Part model, mm, in its own coordinate system. A direction names the side the tool comes from. Coordinates: 2 decimals unless noted, no trailing zeros. Write each loop counter-clockwise with the first axis right and the second up, starting at its lowest first coordinate (ties: lowest second). Pieces come first, ordered by that corner, then holes. Notation, with made-up numbers: (24.5, 6) - (58.5, 6) arc R23 cw to (58.5, 29) - close; hole circle Ø1 at (30, 70.5). An arc over 180 degrees is marked (long way). Use a Markdown table: item, result.
```python
from build123d import *

# Parameters (mm, degrees)
SKETCH_W               = 265
SKETCH_H               = 132.5
PAD_DEPTH              = 23
SKETCH001_W            = 249
SKETCH001_H            = 124.5
POCKET_DEPTH           = 2
SKETCH002_W            = 30
SKETCH002_H            = 30
PAD001_DEPTH           = 2
LINEARPATTERN_COUNT    = 8
LINEARPATTERN_PITCH    = 31
CHAMFER_SIZE           = 3
SKETCH003_W            = 31.42
SKETCH003_H            = 15.71
POCKET001_DEPTH        = 4.8
SKETCH004_W            = 255
SKETCH004_H            = 114.5
POCKET002_DEPTH        = 19
SKETCH005_R            = 7.6
POCKET003_DEPTH        = 2
LINEARPATTERN001_COUNT = 8
LINEARPATTERN001_PITCH = 32.142857
SKETCH006_R            = 7.6
POCKET004_DEPTH        = 2
LINEARPATTERN002_COUNT = 9
LINEARPATTERN002_PITCH = 28.125
SKETCH007_R            = 4.125
SKETCH007_R_2          = 4.025
POCKET005_DEPTH        = 1.8


with BuildPart() as part:
    # Sketch → Pad (new body)
    with BuildSketch(Plane.XY):
        with Locations((0, 66.25)):
            Rectangle(SKETCH_W, SKETCH_H)
    extrude(amount=PAD_DEPTH)

    # Sketch001 (on Face5 of Pad) → Pocket (cut)
    with BuildSketch(Plane(origin=(0, 0, 0), x_dir=(1, 0, 0), z_dir=(0, 0, -1))):
        with Locations((0, -62.25)):
            Rectangle(SKETCH001_W, SKETCH001_H)
    extrude(amount=-POCKET_DEPTH, mode=Mode.SUBTRACT)

    # Sketch002 (on Face10 of Pocket) → Pad001 (join)
    with BuildSketch(Plane(origin=(0, 0, 2), x_dir=(1, 0, 0), z_dir=(0, 0, -1))):
        with Locations((-108.5, -15.5)):
            Rectangle(SKETCH002_W, SKETCH002_H)
        with Locations((-108.5, -46.5)):
            Rectangle(SKETCH002_W, SKETCH002_H)
        with Locations((-108.5, -77.5)):
            Rectangle(SKETCH002_W, SKETCH002_H)
        with Locations((-108.5, -108.5)):
            Rectangle(SKETCH002_W, SKETCH002_H)
    pad001 = extrude(amount=PAD001_DEPTH)

    # LinearPattern: Pad001 ×8
    with Locations(*[(i * LINEARPATTERN_PITCH, 0, 0) for i in range(1, LINEARPATTERN_COUNT)]):
        add(pad001)

    # Chamfer
    chamfer_edges = [part.edges().sort_by_distance(p)[0] for p in [
        (-132.5, 66.25, 0),
        (0, 132.5, 0),
        (132.5, 66.25, 0),
    ]]
    chamfer(chamfer_edges, length=CHAMFER_SIZE)

    # Sketch003 (on Face6 of Chamfer) → Pocket001 (cut)
    with BuildSketch(Plane.XZ):
        with Locations((-86.79, 15.145)):
            Rectangle(SKETCH003_W, SKETCH003_H)
        with Locations((86.79, 15.145)):
            Rectangle(SKETCH003_W, SKETCH003_H)
    extrude(amount=-POCKET001_DEPTH, mode=Mode.SUBTRACT)

    # Sketch004 (on Face4 of Pocket001) → Pocket002 (cut)
    with BuildSketch(Plane.XY.offset(23)):
        with Locations((0, 65.25)):
            Rectangle(SKETCH004_W, SKETCH004_H)
    extrude(amount=-POCKET002_DEPTH, mode=Mode.SUBTRACT)

    # Sketch005 (on Face17 of Pocket002) → Pocket003 (cut)
    with BuildSketch(Plane(origin=(0, 8, 0), x_dir=(-1, 0, 0), z_dir=(0, 1, 0))):
        with Locations((-112.5, 13.5)):
            Circle(SKETCH005_R)
    pocket003 = extrude(amount=-POCKET003_DEPTH, mode=Mode.SUBTRACT)

    # LinearPattern001: Pocket003 ×8
    with Locations(*[(-i * LINEARPATTERN001_PITCH, 0, 0) for i in range(1, LINEARPATTERN001_COUNT)]):
        add(pocket003, mode=Mode.SUBTRACT)

    # Sketch006 (on Face19 of Pocket002) → Pocket004 (cut)
    with BuildSketch(Plane.XZ.offset(-122.5)):
        with Locations((-112.5, 13.5)):
            Circle(SKETCH006_R)
    pocket004 = extrude(amount=-POCKET004_DEPTH, mode=Mode.SUBTRACT)

    # LinearPattern002: Pocket004 ×9
    with Locations(*[(i * LINEARPATTERN002_PITCH, 0, 0) for i in range(1, LINEARPATTERN002_COUNT)]):
        add(pocket004, mode=Mode.SUBTRACT)

    # Sketch007 (on Face4 of LinearPattern002) → Pocket005 (cut)
    with BuildSketch(Plane.XY.offset(23)):
        with Locations((-117.5, 127.5)):
            Circle(SKETCH007_R)
        with Locations((117.5, 127.5)):
            Circle(SKETCH007_R_2)
    extrude(amount=-POCKET005_DEPTH, mode=Mode.SUBTRACT)


solid = part.part
```
Item 1: Which spindle directions (+Z, -Z, +X, -X, +Y, -Y) get a long thin tool onto all of the face, cutting with end or side? Do faces 1 (the face through (117, 128, 21.2)), 2 (the face through (71.08, 2, 15)), 3 (the face through (73.337, 7.014, 10.589)). Say none if no direction does.
From the geometry:
| item | result |
|---|---|
| face 1 | +Z |
| face 2 | +Z, -Y |
| face 3 | none |
Item 2: Two-plate mould, pull along Y, no slides. Class faces 4 (the face through (3.51, 123.49, 6.76)), 5 (the face through (113, 6, 14)), 6 (the face through (77, 15, 0)): pulls with the +Y half, pulls with the -Y half, needs draft (parallel to the pull), parting line crosses it, or undercut.
From the geometry:
| item | result |
|---|---|
| face 4 | undercut |
| face 5 | undercut |
| face 6 | needs draft |
Item 3: Drill centre lines: probe 1 along Y at (x, z) = (-117.5, 22) (3 decimals); probe 2 along X at (y, z) = (109, 4.25); probe 3 along Y at (x, z) = (-64, 4.75). Where is each one in solid material? Low to high.
From the geometry:
| item | result |
|---|---|
| probe 1 | 0 to 8, 122.5 to 123.375, 131.625 to 132.5 |
| probe 2 | -132.5 to -127.5, 127.5 to 132.5 |
| probe 3 | 0 to 8, 122.5 to 132.5 |
Item 4: Drop flat-ended pins along their axis: P1, Ø2, axis at x = 21, z = 0.5, coming from the -Y side; P2, Ø1.5, axis at x = -25.5, y = 81, coming from the +Z side; P3, Ø2, axis at y = 72.5, z = 1.5, coming from the -X side; P4, Ø9.5, axis at x = 117.5, y = 127.5, coming from the +Z side. Give the stop position or say it passes through.
From the geometry:
| item | result |
|---|---|
| P1 | y = 0.5 |
| P2 | z = 4 |
| P3 | x = -132 |
| P4 | z = 23 |
Item 5: Band-saw the part on A-A, the plane x = 68. Give the cut face in (y, z), then the cut area to 4 significant figures.
From the geometry:
| item | result |
|---|---|
| outline | (0, 2) - (0.5, 2) - (0.5, 0) - (30.5, 0) - (30.5, 2) - (31.5, 2) - (31.5, 0) - (61.5, 0) - (61.5, 2) - (62.5, 2) - (62.5, 0) - (92.5, 0) - (92.5, 2) - (93.5, 2) - (93.5, 0) - (123.5, 0) - (123.5, 2) - (124.5, 2) - (124.5, 0) - (129.5, 0) - (132.5, 3) - (132.5, 23) - (122.5, 23) - (122.5, 4) - (8, 4) - (8, 23) - (0, 23) - close |
| area | 858.5 mm^2 |
